Verification items for the finished model (mm, model axes). A direction names the side the tool comes from. Round coordinates to 2 decimals unless told otherwise and drop trailing zeros. Order: outer loops, then holes, each group sorted by start corner. A loop starts at its lowest first (then second) coordinate and runs counter-clockwise, first axis right, second up. Notation, with made-up numbers: (-17, -11.5) -> (4, -11.5) arc R32 cw to (4, 27.5) -> close; hole circle Ø6 at (-32, 76). An arc over 180 degrees is marked (long way). Return JSON: item names as keys, results as strings. Group by question number.
1) Section check B-B on z = 5.25. Enter the section's corners in (x, y) (3 decimals), plus the area to 3 significant figures.
2) Draft check along X on faces 1 (the flat face through (6.985, 18.896, 9.392)), 2 (the flat face through (-27.58, 29.24, 9.39)), 3 (the flat face through (1, -19.05, 7)). Enter one of: pulls with the +X half, pulls with the -X half, needs draft (parallel to the pull), parting line crosses it, or undercut.
3) Section check A-A on x = 0. Enter the section's corners in (y, z) (3 decimals), plus the area to 3 significant figures.
4) Section check D-D on y = 14.5. Enter the section's corners in (x, z), plus the area to 3 significant figures.
5) Section check C-C on y = -12.5. Enter the section's corners in (x, z) (3 decimals).
6) Scan lines: L1, parallel to Z at x = 0, y = 0 (3 decimals); L2, parallel to Y at x = 4, z = 4 (3 decimals); L3, parallel to Z at x = -1, y = -8.5. Record each from-to range of solid material in increasing order.
7) Depth check by flat-ended pin: pin 1 (4 mm diameter, centred on x = -17, z = 12.5, fed in from +Y); pin 2 (1 mm diameter, centred on x = 20, z = 4, fed in from +Y); pin 3 (4 mm diameter, centred on x = 0, z = 9.525, fed in from -Y). Enter the tip coordinate at first touch or a pass-through.
8) Tool access check on faces 4 (the flat face through (-6.35, -11, 9)), 5 (the flat face through (0, 8, 0)), 6 (the flat face through (26.31, 32.66, 9.39)), 7 (the cylindrical face through (-0.551, -6.528, 7.045)), 8 (the flat face through (6.35, -11, 9)). Record the directions out of +Z, -Z, +X, -X, +Y, -Y that give a thin tool (end or side, any length) a straight path to the whole face; none if there is none.
```python
from build123d import *

# Parameters (mm, degrees)
F1_DEPTH = 19.05
F2_R     = 2.54
F3_DEPTH = 25.4


with BuildPart() as f1:
    # F0 (on Top) → F1 (new body)
    with BuildSketch(Plane.XY):
        with BuildLine():
            Line((6.35, 0), (0, 0))
            Line((0, 0), (0, -6.35))
            ThreePointArc((0, -6.35), (2.7507484386, -5.7232755505), (4.95851694, -3.966813552))
            ThreePointArc((4.95851694, -3.966813552), (5.9920398267, -2.1018940781), (6.35, 0))
        make_face()
        with BuildLine():
            Line((0, -6.35), (0, 0))
            Line((0, 0), (-6.35, 0))
            ThreePointArc((-6.35, 0), (-5.9920398267, -2.1018940781), (-4.95851694, -3.966813552))
            ThreePointArc((-4.95851694, -3.966813552), (-2.7507484386, -5.7232755505), (0, -6.35))
        make_face()
        with BuildLine():
            Line((0, 0), (-4.0659838908, 5.0824798635))
            Line((-4.0659838908, 5.0824798635), (-4.95851694, 3.966813552))
            ThreePointArc((-4.95851694, 3.966813552), (-5.9920398267, 2.1018940781), (-6.35, 0))
            Line((-6.35, 0), (0, 0))
        make_face()
        with BuildLine():
            Line((4.0659838908, 5.0824798635), (0, 0))
            Line((0, 0), (6.35, 0))
            ThreePointArc((6.35, 0), (5.9920398267, 2.1018940781), (4.95851694, 3.966813552))
            Line((4.95851694, 3.966813552), (4.0659838908, 5.0824798635))
        make_face()
        Polygon((0, 10.1649597269), (-4.0659838908, 5.0824798635), (0, 0), (4.0659838908, 5.0824798635), align=None)
        with BuildLine():
            Line((-4.0659838908, 5.0824798635), (-12.7, 15.875))
            Line((-12.7, 15.875), (-23.0199118688, 28.774889836))
            Line((-23.0199118688, 28.774889836), (-25.4, 31.75))
            Line((-25.4, 31.75), (-27.1960512242, 33.5460512242))
            Line((-27.1960512242, 33.5460512242), (-27.9784288088, 24.8080762841))
            Line((-27.9784288088, 24.8080762841), (-6.35, -2.2274597269))
            Line((-6.35, -2.2274597269), (-6.35, 0))
            ThreePointArc((-6.35, 0), (-5.9920398267, 2.1018940781), (-4.95851694, 3.966813552))
            Line((-4.95851694, 3.966813552), (-4.0659838908, 5.0824798635))
        make_face()
        Polygon((-4.5680322185, 15.875), (-12.7, 15.875), (-4.0659838908, 5.0824798635), (0, 10.1649597269), align=None)
        Polygon((4.5680322185, 15.875), (0, 10.1649597269), (4.0659838908, 5.0824798635), (12.7, 15.875), align=None)
        Polygon((4.5680322185, 15.875), (-4.5680322185, 15.875), (0, 10.1649597269), align=None)
        with BuildLine():
            Line((12.7, 15.875), (4.0659838908, 5.0824798635))
            Line((4.0659838908, 5.0824798635), (4.95851694, 3.966813552))
            ThreePointArc((4.95851694, 3.966813552), (5.9920398267, 2.1018940781), (6.35, 0))
            Line((6.35, 0), (6.35, -2.2274597269))
            Line((6.35, -2.2274597269), (27.9784288088, 24.8080762841))
            Line((27.9784288088, 24.8080762841), (27.1960512242, 33.5460512242))
            Line((27.1960512242, 33.5460512242), (25.4, 31.75))
            Line((25.4, 31.75), (23.0199118688, 28.774889836))
            Line((23.0199118688, 28.774889836), (12.7, 15.875))
        make_face()
        Polygon((9.3344051145, 21.8329661201), (4.5680322185, 15.875), (12.7, 15.875), (23.0199118688, 28.774889836), align=None)
        Polygon((-23.0199118688, 28.774889836), (-12.7, 15.875), (-4.5680322185, 15.875), (-9.3344051145, 21.8329661201), align=None)
        Polygon((23.6039487758, 33.5460512242), (23.0199118688, 28.774889836), (25.4, 31.75), align=None)
        Polygon((-25.4, 31.75), (-23.0199118688, 28.774889836), (-23.6039487758, 33.5460512242), align=None)
        with BuildLine():
            ThreePointArc((-4.95851694, -3.966813552), (-5.9920398267, -2.1018940781), (-6.35, 0))
            Line((-6.35, 0), (-6.35, -2.2274597269))
            Line((-6.35, -2.2274597269), (-4.95851694, -3.966813552))
        make_face()
        with BuildLine():
            Line((6.35, -2.2274597269), (6.35, 0))
            ThreePointArc((6.35, 0), (5.9920398267, -2.1018940781), (4.95851694, -3.966813552))
            Line((4.95851694, -3.966813552), (6.35, -2.2274597269))
        make_face()
        with BuildLine():
            ThreePointArc((4.95851694, -3.966813552), (2.7507484386, -5.7232755505), (0, -6.35))
            Line((0, -6.35), (0, -19.05))
            Line((0, -19.05), (6.35, -19.05))
            Line((6.35, -19.05), (6.35, -2.2274597269))
            Line((6.35, -2.2274597269), (4.95851694, -3.966813552))
        make_face()
        with BuildLine():
            Line((0, -19.05), (0, -6.35))
            ThreePointArc((0, -6.35), (-2.7507484386, -5.7232755505), (-4.95851694, -3.966813552))
            Line((-4.95851694, -3.966813552), (-6.35, -2.2274597269))
            Line((-6.35, -2.2274597269), (-6.35, -19.05))
            Line((-6.35, -19.05), (0, -19.05))
        make_face()
    extrude(amount=F1_DEPTH)

    # F2 (on face) → F3 (cut)
    with BuildSketch(Plane.XZ.offset(19.05)):
        with Locations((0, 9.525)):
            Circle(F2_R)
    extrude(amount=-F3_DEPTH, mode=Mode.SUBTRACT)


solid = f1.part
```
Check result:
{
 "1": {"outline": "(-27.978, 24.808) -> (-6.35, -2.227) -> (-6.35, -19.05) -> (6.35, -19.05) -> (6.35, -2.227) -> (27.978, 24.808) -> (27.196, 33.546) -> (25.4, 31.75) -> (23.604, 33.546) -> (23.02, 28.775) -> (9.334, 21.833) -> (4.568, 15.875) -> (-4.568, 15.875) -> (-9.334, 21.833) -> (-23.02, 28.775) -> (-23.604, 33.546) -> (-25.4, 31.75) -> (-27.196, 33.546) -> close", "area": "1,090 mm^2"},
 "2": {"face 1": "undercut", "face 2": "pulls with the -X half", "face 3": "needs draft"},
 "3": {"outline": "(-19.05, 0) -> (15.875, 0) -> (15.875, 19.05) -> (-19.05, 19.05) -> (-19.05, 12.065) -> (6.35, 12.065) -> (6.35, 6.985) -> (-19.05, 6.985) -> close", "area": "536 mm^2"},
 "4": {"outline": "(-19.73, 0) -> (19.73, 0) -> (19.73, 19.05) -> (-19.73, 19.05) -> close", "area": "752 mm^2"},
 "5": {"outline": "(-6.35, 0) -> (6.35, 0) -> (6.35, 19.05) -> (-6.35, 19.05) -> close; hole circle Ø5.08 at (0, 9.525)"},
 "6": {"L1": "0 to 6.985, 12.065 to 19.05", "L2": "-19.05 to 15.875", "L3": "0 to 7.19, 11.86 to 19.05"},
 "7": {"pin 1": "y = 26.74", "pin 2": "y = 27.5", "pin 3": "y = 6.35"},
 "8": {"face 4": "+Z, -Z, -X, -Y", "face 5": "-Z, +X, -X, +Y, -Y", "face 6": "+Z, -Z, +Y", "face 7": "-Y", "face 8": "+Z, -Z, +X, -Y"}
}
